Geometry: final body of the model. Coordinates: model frame, mm. Give positions to 0.01 mm unless a question says otherwise; leave off trailing zeros. Write each loop counter-clockwise with the first axis right and the second up, starting at its lowest first coordinate (ties: lowest second). Pieces come first, ordered by that corner, then holes. Notation, with made-up numbers: (66.25, 88.5) -> (125.25, 88.5) arc R12 ccw to (125.25, 98.5) -> close; hole circle Ø5 at (89.5, 40). An arc over 180 degrees is marked (long way). Answer as a JSON object with one key per item and string values. Group by question number.
(1) Section query A-A on z = 220.5. Output: boundary loops of the cut face in (x, y), plus the area to 3 significant figures.
(2) Section query B-B on x = 2. Output: boundary loops of the cut face in (y, z), plus the area to 3 significant figures.
(3) Contact query for flat-ended pins moving along their axis: pin 1 Ø0.5 at (x, y) = (-1.5, -3) entering from +Z; pin 2 Ø1.5 at (x, z) = (-3, 404.5) entering from -Y; pin 3 Ø8 at (y, z) = (5.5, 365.5) entering from +X. Output: stop coordinate, or through.
(4) Section query C-C on y = 5.25. Output: boundary loops of the cut face in (x, z).
(5) Material intervals for probe 1 along Y at (x, z) = (4.5, 233); probe 2 along Y at (x, z) = (3.25, 40); probe 3 along X at (y, z) = (2.5, 134), sorted ascending.
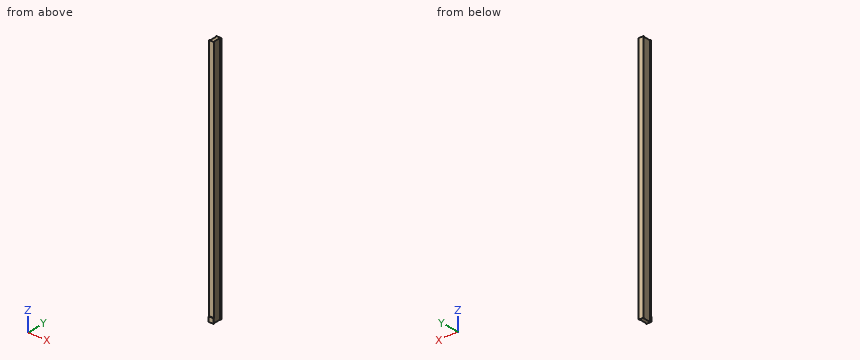
from build123d import *

# Parameters (mm, degrees)
F1_DEPTH = 500.5
F2_W     = 10
F2_H     = 10
F3_DEPTH = 1


with BuildPart() as f1:
    # F0 (on Top) → F1 (new body)
    with BuildSketch(Plane.XY):
        Polygon((5, 15.438399), (-5, 15.438399), (-5, 14.438399), (-3.67, 14.438399), (-3.67, -1.142601), (-5, -1.142601), (-5, -2.142601), (5, -2.142601), (5, -1.142601), (3.67, -1.142601), (3.67, 14.438399), (5, 14.438399), align=None)
    extrude(amount=F1_DEPTH)

    # F2 (on face) → F3 (join)
    with BuildSketch(Plane.XZ.offset(2.142601)):
        with Locations((0, 5)):
            Rectangle(F2_W, F2_H)
    extrude(amount=F3_DEPTH)


solid = f1.part
Answer list:
{
 "1": {"outline": "(-5, -2.14) -> (5, -2.14) -> (5, -1.14) -> (3.67, -1.14) -> (3.67, 14.44) -> (5, 14.44) -> (5, 15.44) -> (-5, 15.44) -> (-5, 14.44) -> (-3.67, 14.44) -> (-3.67, -1.14) -> (-5, -1.14) -> close", "area": "134 mm2"},
 "2": {"outline": "(-3.14, 0) -> (15.44, 0) -> (15.44, 500.5) -> (-2.14, 500.5) -> (-2.14, 10) -> (-3.14, 10) -> close", "area": "8,810 mm2"},
 "3": {"pin 1": "z = 10", "pin 2": "y = -2.14", "pin 3": "x = 3.67"},
 "4": {"outline": "(-3.67, 0) -> (3.67, 0) -> (3.67, 500.5) -> (-3.67, 500.5) -> close"},
 "5": {"probe 1": "-2.14 to -1.14, 14.44 to 15.44", "probe 2": "-2.14 to 15.44", "probe 3": "-3.67 to 3.67"}
}
